Part model, mm, in its own coordinate system. Round coordinates to 2 decimals unless told otherwise and drop trailing zeros. Loops run counter-clockwise (first coordinate to the right, second up) from the corner with the lowest first, then second, coordinate; pieces in that order, holes last. Notation, with made-up numbers: (23.5, 50) -> (30.5, 50) arc R21 ccw to (30.5, 76) -> close; hole circle Ø11 at (67.5, 0). An arc over 180 degrees is marked (long way). Use a Markdown table: item, result. Add a question column.
Item 1: Two-plate mould, pull along Y, no slides. Class faces 1 (the face through (37, 281, 3)), 2 (the face through (54, 277.55, 1)), 3 (the face through (36, 298.55, 1)): pulls with the +Y half, pulls with the -Y half, needs draft (parallel to the pull), parting line crosses it, or undercut.
Item 2: Cut at A-A, the plane x = 27.5. List the corners of the cut face in (y, z).
Item 3: Cut at B-B, the plane y = 276.5. State how many separate pieces and enclosed holes the cut face has, plus the area to 3 significant figures.
Item 4: Flat gauge pin, fed straight in: pin 1 (1.5 mm diameter, centred on x = 54.5, y = 268.5, fed in from -Z). Where does the tip first touch, or does it go through?
Item 5: Probe line 1 (Y direction, x = 55, z = 1.2); line 2 (Y direction, x = 9, z = 1.65); line 3 (X direction, y = 255.5, z = 1.8). List the from-to ranges inside material, lowest first. Write a range as [from, to].
```python
from build123d import *

# Parameters (mm, degrees)
MODEL_W                 = 3
MODEL_H                 = 3
SALIENTE_EXTRUIR1_DEPTH = 3


with BuildPart() as part:
    # Model → Saliente-Extruir1 (new body)
    with BuildSketch(Plane.XY):
        with BuildLine():
            Line((9.385930567, 298.549610222), (63.385930567, 298.549610222))
            ThreePointArc((63.385930567, 298.549610222), (66.567911083, 297.231590737), (67.885930567, 294.049610222))
            Line((67.885930567, 294.049610222), (67.885930567, 258.049610222))
            ThreePointArc((67.885930567, 258.049610222), (66.567911083, 254.867629706), (63.385930567, 253.549610222))
            Line((63.385930567, 253.549610222), (9.385930567, 253.549610222))
            ThreePointArc((9.385930567, 253.549610222), (6.203950052, 254.867629706), (4.885930567, 258.049610222))
            Line((4.885930567, 258.049610222), (4.885930567, 294.049610222))
            ThreePointArc((4.885930567, 294.049610222), (6.203950052, 297.231590737), (9.385930567, 298.549610222))
        make_face()
        with Locations((9.385930567, 294.049610222)):
            Rectangle(MODEL_W, MODEL_H, mode=Mode.SUBTRACT)
        with Locations((18.385930567, 294.049610222)):
            Rectangle(MODEL_W, MODEL_H, mode=Mode.SUBTRACT)
        with Locations((27.385930567, 294.049610222)):
            Rectangle(MODEL_W, MODEL_H, mode=Mode.SUBTRACT)
        with Locations((54.385930567, 294.049610222)):
            Rectangle(MODEL_W, MODEL_H, mode=Mode.SUBTRACT)
        with Locations((63.385930567, 294.049610222)):
            Rectangle(MODEL_W, MODEL_H, mode=Mode.SUBTRACT)
        with Locations((9.385930567, 258.049610222)):
            Rectangle(MODEL_W, MODEL_H, mode=Mode.SUBTRACT)
        with Locations((18.385930567, 258.049610222)):
            Rectangle(MODEL_W, MODEL_H, mode=Mode.SUBTRACT)
        with Locations((27.385930567, 258.049610222)):
            Rectangle(MODEL_W, MODEL_H, mode=Mode.SUBTRACT)
        with Locations((54.385930567, 258.049610222)):
            Rectangle(MODEL_W, MODEL_H, mode=Mode.SUBTRACT)
        with Locations((63.385930567, 258.049610222)):
            Rectangle(MODEL_W, MODEL_H, mode=Mode.SUBTRACT)
        with Locations((9.385930567, 267.049610222)):
            Rectangle(MODEL_W, MODEL_H, mode=Mode.SUBTRACT)
        with Locations((18.385930567, 267.049610222)):
            Rectangle(MODEL_W, MODEL_H, mode=Mode.SUBTRACT)
        with Locations((27.385930567, 267.049610222)):
            Rectangle(MODEL_W, MODEL_H, mode=Mode.SUBTRACT)
        with Locations((54.385930567, 267.049610222)):
            Rectangle(MODEL_W, MODEL_H, mode=Mode.SUBTRACT)
        with Locations((63.385930567, 267.049610222)):
            Rectangle(MODEL_W, MODEL_H, mode=Mode.SUBTRACT)
        with Locations((36.385930567, 294.049610222)):
            Rectangle(MODEL_W, MODEL_H, mode=Mode.SUBTRACT)
        with Locations((45.385930567, 294.049610222)):
            Rectangle(MODEL_W, MODEL_H, mode=Mode.SUBTRACT)
        with Locations((36.385930567, 258.049610222)):
            Rectangle(MODEL_W, MODEL_H, mode=Mode.SUBTRACT)
        with Locations((45.385930567, 258.049610222)):
            Rectangle(MODEL_W, MODEL_H, mode=Mode.SUBTRACT)
        with Locations((36.385930567, 267.049610222)):
            Rectangle(MODEL_W, MODEL_H, mode=Mode.SUBTRACT)
        with Locations((45.385930567, 267.049610222)):
            Rectangle(MODEL_W, MODEL_H, mode=Mode.SUBTRACT)
        with Locations((9.385930567, 276.049610222)):
            Rectangle(MODEL_W, MODEL_H, mode=Mode.SUBTRACT)
        with Locations((18.385930567, 276.049610222)):
            Rectangle(MODEL_W, MODEL_H, mode=Mode.SUBTRACT)
        with Locations((27.385930567, 276.049610222)):
            Rectangle(MODEL_W, MODEL_H, mode=Mode.SUBTRACT)
        with Locations((54.385930567, 276.049610222)):
            Rectangle(MODEL_W, MODEL_H, mode=Mode.SUBTRACT)
        with Locations((63.385930567, 276.049610222)):
            Rectangle(MODEL_W, MODEL_H, mode=Mode.SUBTRACT)
        with Locations((9.385930567, 285.049610222)):
            Rectangle(MODEL_W, MODEL_H, mode=Mode.SUBTRACT)
        with Locations((18.385930567, 285.049610222)):
            Rectangle(MODEL_W, MODEL_H, mode=Mode.SUBTRACT)
        with Locations((27.385930567, 285.049610222)):
            Rectangle(MODEL_W, MODEL_H, mode=Mode.SUBTRACT)
        with Locations((54.385930567, 285.049610222)):
            Rectangle(MODEL_W, MODEL_H, mode=Mode.SUBTRACT)
        with Locations((63.385930567, 285.049610222)):
            Rectangle(MODEL_W, MODEL_H, mode=Mode.SUBTRACT)
        with Locations((36.385930567, 276.049610222)):
            Rectangle(MODEL_W, MODEL_H, mode=Mode.SUBTRACT)
        with Locations((45.385930567, 276.049610222)):
            Rectangle(MODEL_W, MODEL_H, mode=Mode.SUBTRACT)
        with Locations((36.385930567, 285.049610222)):
            Rectangle(MODEL_W, MODEL_H, mode=Mode.SUBTRACT)
        with Locations((45.385930567, 285.049610222)):
            Rectangle(MODEL_W, MODEL_H, mode=Mode.SUBTRACT)
    extrude(amount=SALIENTE_EXTRUIR1_DEPTH)


solid = part.part
```
A:
| question | item | result |
|---|---|---|
| 1 | face 1 | needs draft |
| 1 | face 2 | undercut |
| 1 | face 3 | pulls with the +Y half |
| 2 | outline | (253.55, 0) -> (256.55, 0) -> (256.55, 3) -> (253.55, 3) -> close; (259.55, 0) -> (265.55, 0) -> (265.55, 3) -> (259.55, 3) -> close; (268.55, 0) -> (274.55, 0) -> (274.55, 3) -> (268.55, 3) -> close; (277.55, 0) -> (283.55, 0) -> (283.55, 3) -> (277.55, 3) -> close; (286.55, 0) -> (292.55, 0) -> (292.55, 3) -> (286.55, 3) -> close; (295.55, 0) -> (298.55, 0) -> (298.55, 3) -> (295.55, 3) -> close |
| 3 | separate pieces | 8 |
| 3 | enclosed holes | 0 |
| 3 | area | 126 mm^2 |
| 4 | pin 1 | stops at z = 0 |
| 5 | line 1 | y = [253.55, 256.55], [259.55, 265.55], [268.55, 274.55], [277.55, 283.55], [286.55, 292.55], [295.55, 298.55] |
| 5 | line 2 | y = [253.57, 256.55], [259.55, 265.55], [268.55, 274.55], [277.55, 283.55], [286.55, 292.55], [295.55, 298.53] |
| 5 | line 3 | x = [5.68, 67.09] |
